from build123d import *

# Parameters (mm, degrees)
F0_W     = 50.8
F0_H     = 50.8
F1_DEPTH = 63.5
F2_R     = 50.79999


# Not quite as in the source:
# - a fillet or chamfer is up to 0.001 mm smaller than in the source, because OpenCascade refuses the exact size


with BuildPart() as f1:
    # F0 (on Top) → F1 (new body, symmetric)
    with BuildSketch(Plane.XY):
        Rectangle(F0_W, F0_H)
    extrude(amount=F1_DEPTH, both=True)

    # F2 (radius 50.8 in the source; OpenCascade refuses exactly that, so slightly less here)
    f2_edges = [f1.edges().sort_by_distance(p)[0] for p in [
        (25.4, 0, 63.5),
    ]]
    fillet(f2_edges, radius=F2_R)


solid = f1.part
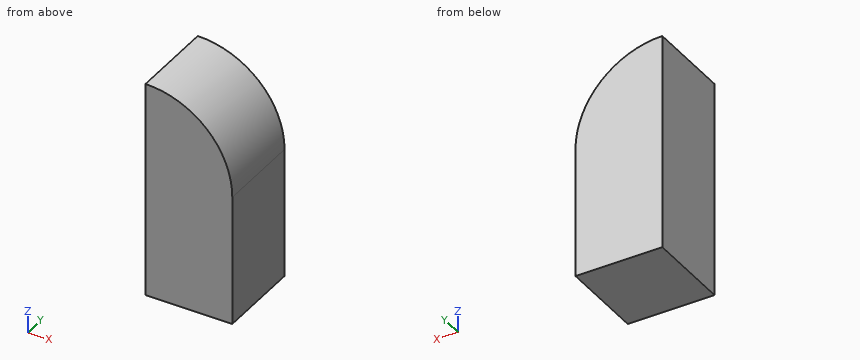
Work out the finished part from the listing and answer in its coordinate system (mm). Give positions to 0.01 mm unless a question says otherwise; leave off trailing zeros. Loops run counter-clockwise (first coordinate to the right, second up) from the corner with the lowest first, then second, coordinate; pieces in that order, holes last. Notation, with made-up numbers: (-22, 1.25) -> (13, 1.25) arc R28 ccw to (13, 35.25) -> close; hole circle Ø7 at (17.25, 72). An arc over 180 degrees is marked (long way). Use a Markdown table: item, result. Add a question column.
1. Section B-B on x = 21.5 is taken. Determine the outline of the cut face in (y, z), and give its area (3 significant figures).
2. Find the intervals of material crossed by probe 1 along Z at (x, y) = (13, 3); probe 2 along Z at (x, y) = (5.5, -20.5); probe 3 along X at (y, z) = (-17, 33.5), in increasing order.
3. Section C-C on z = 49 is taken. Determine the outline of the cut face in (x, y).
4. Flat-ended cylindrical pins translate along their axes: pin 1 Ø1.5 at (x, y) = (4, -11) entering from +Z; pin 2 Ø4 at (y, z) = (4, 16.5) entering from +X. Find the tip coordinate at first contact, or state that the pin passes through.
Results below:
| question | item | result |
|---|---|---|
| 1 | outline | (-25.4, -63.5) -> (25.4, -63.5) -> (25.4, 32.22) -> (-25.4, 32.22) -> close |
| 1 | area | 4,860 mm^2 |
| 2 | probe 1 | z = -63.5 to 45.96 |
| 2 | probe 2 | z = -63.5 to 53.02 |
| 2 | probe 3 | x = -25.4 to 20.95 |
| 3 | outline | (-25.4, -25.4) -> (10.14, -25.4) -> (10.14, 25.4) -> (-25.4, 25.4) -> close |
| 4 | pin 1 | stops at z = 54.65 |
| 4 | pin 2 | stops at x = 25.37 |
